from build123d import *

# Parameters (mm, degrees)
F0_R     = 1.5875
F1_DEPTH = 3.048


with BuildPart() as f1:
    # F0 (on Top) → F1 (new body)
    with BuildSketch(Plane.XY):
        with BuildLine():
            ThreePointArc((1.5875, 0), (-1.1225320151, -1.1225320151), (0, 1.5875))
            Line((0, 1.5875), (0, 9.525))
            ThreePointArc((0, 9.525), (-7.063929059, 6.3895642457), (-9.4772553384, -0.9525))
            ThreePointArc((-9.4772553384, -0.9525), (-6.2623833816, -7.1769199091), (0.3401785714, -9.5189234444))
            ThreePointArc((0.3401785714, -9.5189234444), (6.8544082857, -6.6138273378), (9.525, 0))
            Line((9.525, 0), (1.5875, 0))
        make_face()
        with BuildLine():
            ThreePointArc((-9.4772553384, -0.9525), (-7.063929059, 6.3895642457), (0, 9.525))
            Line((0, 9.525), (0, 47.625))
            ThreePointArc((0, 47.625), (-10.6492737428, 51.7267849017), (-15.7954255641, 61.9125))
            Line((-15.7954255641, 61.9125), (-9.4772553384, -0.9525))
        make_face()
        with BuildLine():
            Line((0, 47.625), (0, 9.525))
            ThreePointArc((0, 9.525), (6.7351920908, 6.7351920908), (9.525, 0))
            Line((9.525, 0), (36.5125, 0))
            ThreePointArc((36.5125, 0), (38.9380895153, 5.7116327839), (44.7324052746, 7.9324746146))
            Line((44.7324052772, 7.9324746877), (18.9676000005, 8.8532337108))
            ThreePointArc((18.9676000005, 8.8532337108), (13.2611998974, 11.5713591498), (11.3411865923, 17.5933818124))
            Line((11.3411865923, 17.5933818124), (15.7954255641, 61.9125))
            ThreePointArc((15.7954255641, 61.9125), (10.6492737428, 51.7267849017), (0, 47.625))
        make_face()
        with BuildLine():
            Line((36.5125, 0), (9.525, 0))
            ThreePointArc((9.525, 0), (6.8544082857, -6.6138273378), (0.3401785714, -9.5189234444))
            Line((0.3401785714, -9.5189234444), (44.7324052772, -7.9324746877))
            ThreePointArc((44.7324052746, -7.9324746146), (38.9380895153, -5.7116327839), (36.5125, 0))
        make_face()
        with BuildLine():
            ThreePointArc((-15.7954255641, 61.9125), (-10.6492737428, 51.7267849017), (0, 47.625))
            Line((0, 47.625), (0, 61.9125))
            ThreePointArc((0, 61.9125), (-1.5875, 63.5), (0, 65.0875))
            Line((0, 65.0875), (0, 79.375))
            ThreePointArc((0, 79.375), (-10.4912828548, 75.4142187767), (-15.7474569047, 65.5082893304))
            ThreePointArc((-15.7474569047, 65.5082893304), (-15.8735876171, 63.7117573215), (-15.7954255641, 61.9125))
        make_face()
        with BuildLine():
            Line((0, 61.9125), (0, 47.625))
            ThreePointArc((0, 47.625), (10.6492737428, 51.7267849017), (15.7954255641, 61.9125))
            ThreePointArc((15.7954255641, 61.9125), (15.8550939106, 62.7052534459), (15.875, 63.5))
            ThreePointArc((15.875, 63.5), (15.8430821396, 64.5061676396), (15.7474569047, 65.5082893304))
            ThreePointArc((15.7474569047, 65.5082893304), (10.4912828548, 75.4142187767), (0, 79.375))
            Line((0, 79.375), (0, 65.0875))
            ThreePointArc((0, 65.0875), (1.1225320151, 64.6225320151), (1.5875, 63.5))
            ThreePointArc((1.5875, 63.5), (1.1225320151, 62.3774679849), (0, 61.9125))
        make_face()
        with BuildLine():
            ThreePointArc((44.7324052746, 7.9324746146), (38.9380895153, 5.7116327839), (36.5125, 0))
            Line((36.5125, 0), (42.8625, 0))
            ThreePointArc((42.8625, 0), (43.4321989692, 1.2182927857), (44.7324052746, 1.5621790905))
            Line((44.7324052746, 1.5621790905), (44.7324052746, 7.9324746146))
        make_face()
        with BuildLine():
            Line((42.8625, 0), (36.5125, 0))
            ThreePointArc((36.5125, 0), (38.9380895153, -5.7116327839), (44.7324052746, -7.9324746146))
            Line((44.7324052746, -7.9324746146), (44.7324052746, -1.5621790905))
            ThreePointArc((44.7324052746, -1.5621790905), (43.4321989692, -1.2182927857), (42.8625, 0))
        make_face()
        with BuildLine():
            ThreePointArc((44.7334821429, 7.9324362036), (44.7329437094, 7.9324554274), (44.7324052746, 7.9324746146))
            Line((44.7324052746, 7.9324746146), (44.7324052746, 1.5621790905))
            ThreePointArc((44.7324052746, 1.5621790905), (45.6682927857, 1.0178010308), (46.0375, 0))
            ThreePointArc((46.0375, 0), (45.6682927857, -1.0178010308), (44.7324052746, -1.5621790905))
            Line((44.7324052746, -1.5621790905), (44.7324052746, -7.9324746146))
            ThreePointArc((44.7324052746, -7.9324746146), (44.7329437094, -7.9324554274), (44.7334821429, -7.9324362036))
            ThreePointArc((44.7334821429, -7.9324362036), (50.1620069047, -5.5115227815), (52.3875, 0))
            ThreePointArc((52.3875, 0), (50.1620069047, 5.5115227815), (44.7334821429, 7.9324362036))
        make_face()
        with BuildLine():
            Line((-9.525, 114.3), (-15.7474569047, 65.5082893304))
            ThreePointArc((-15.7474569047, 65.5082893304), (-10.4912828548, 75.4142187767), (0, 79.375))
            Line((0, 79.375), (0, 104.775))
            ThreePointArc((0, 104.775), (-6.7351920908, 107.5648079092), (-9.525, 114.3))
        make_face()
        with Locations((-3.39970598, 100.0252)):
            Circle(F0_R, mode=Mode.SUBTRACT)
        with BuildLine():
            Line((0, 104.775), (0, 79.375))
            ThreePointArc((0, 79.375), (10.4912828548, 75.4142187767), (15.7474569047, 65.5082893304))
            Line((15.7474569047, 65.5082893304), (9.525, 114.3))
            ThreePointArc((9.525, 114.3), (6.7351920908, 107.5648079092), (0, 104.775))
        make_face()
        with BuildLine():
            ThreePointArc((9.525, 114.3), (0, 123.825), (-9.525, 114.3))
            ThreePointArc((-9.525, 114.3), (-6.7351920908, 107.5648079092), (0, 104.775))
            ThreePointArc((0, 104.775), (6.7351920908, 107.5648079092), (9.525, 114.3))
        make_face()
        with BuildLine():
            ThreePointArc((1.5875, 114.3), (1.1225320151, 113.1774679849), (0, 112.7125))
            ThreePointArc((0, 112.7125), (-1.1225320151, 115.4225320151), (1.5875, 114.3))
        make_face(mode=Mode.SUBTRACT)
        with BuildLine():
            Line((0, 9.525), (0, 1.5875))
            ThreePointArc((0, 1.5875), (1.1225320151, 1.1225320151), (1.5875, 0))
            Line((1.5875, 0), (9.525, 0))
            ThreePointArc((9.525, 0), (6.7351920908, 6.7351920908), (0, 9.525))
        make_face()
    extrude(amount=F1_DEPTH)


solid = f1.part
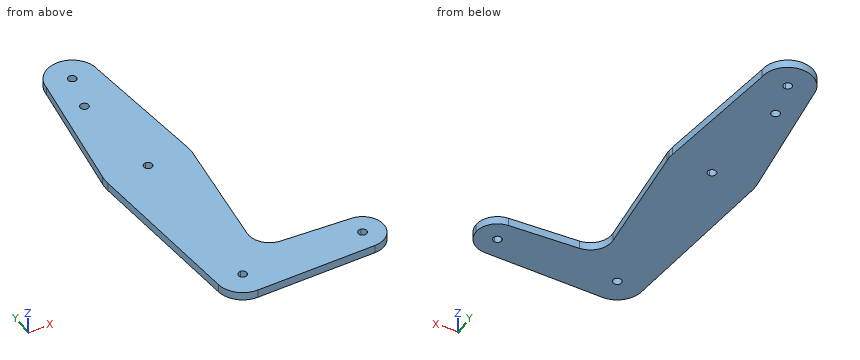
Geometry: final body of the model. Coordinates: model frame, mm. Coordinates: 2 decimals unless noted, no trailing zeros. Loops run counter-clockwise (first coordinate to the right, second up) from the corner with the lowest first, then second, coordinate; pieces in that order, holes last. Notation, with made-up numbers: (58, 37) - (114, 37) arc R18 cw to (114, 71) - close; hole circle Ø8 at (55.25, 53.5). An arc over 180 degrees is marked (long way). Put each result on its own line as item: value. Start each with the question number.
Q1. Pin query (flat end, axial travel): pin 1 Ø1 at (x, z) = (24.5, 2.5) entering from +Y; pin 2 Ø1.5 at (y, z) = (93, 2) entering from -X; pin 3 Ø1.5 at (y, z) = (47.5, 2.5) entering from -X. Return the tip coordinate at first contact, or that it passes through.
Q2. Cut plane B-B, the plane x = 36. Return loops of the section in (y, z).
Q3. Line query: line 1 (Y direction, x = 0, z = 1.75) (1 decimal); line 2 (Y direction, x = 1, z = 1.65); line 3 (X direction, y = 114.3, z = 1.35) (1 decimal). Output: solid intervals per line, ascending.
Q4. Cut plane C-C, the plane y = 51. Return loops of the section in (x, z).
Q5. Cut plane A-A, the plane z = 1.75. Give the number of separate pieces and of enclosed holes in the cut face, and give its area (3 significant figures).
Filled sheet:
1. pin 1: y = 8.67
1. pin 2: x = -12.34
1. pin 3: x = -14.42
2. outline: (-8.24, 0) - (8.24, 0) - (8.24, 3.05) - (-8.24, 3.05) - close
3. line 1: -9.5 to -1.6, 1.6 to 61.9, 65.1 to 112.7, 115.9 to 123.8
3. line 2: -9.5 to -1.23, 1.23 to 62.27, 64.73 to 113.07, 115.53 to 123.77
3. line 3: -9.5 to -1.6, 1.6 to 9.5
4. outline: (-14.7, 0) - (14.7, 0) - (14.7, 3.05) - (-14.7, 3.05) - close
5. separate pieces: 1
5. enclosed holes: 5
5. area: 3,890 mm²
